Could you check a few things on this drawing? It's one solid part, dimensions in mm from its lowest x, y, z. Coordinates: 2 decimals unless noted, no trailing zeros. Loops run counter-clockwise (first coordinate to the right, second up) from the corner with the lowest first, then second, coordinate; pieces in that order, holes last. Notation, with made-up numbers: M 14,17.25 L 30,17.25 A19 cw 30,31.25 Z; hole C -13.5,19.25 d8. An arc over 180 degrees is marked long. Use one line per item in the form item = value. Start each with the question number.
(1) Imagine slicing it at C-C, the plane y = 7.5. Please give me the cut outline in (x, z) (1 decimal).
(2) Please list where these lines run through material, in increasing order: L1, parallel to Y at x = 16, z = 2.25; L2, parallel to Y at x = 16, z = 4.5; L3, parallel to X at y = 17.5, z = 3.
(3) Thinking about a two-plate mould opening in Y: for the marked faces 1, 2 and 3, which applies, +Y half, -Y half, draft (parallel to the pull), parting line (faces both ways), or undercut?
(4) Imagine slicing it at A-A, the plane y = 16. Please give me the cut outline in (x, z).
(5) Will these pins go through, and if not, where does the flat tip stop? P1, Ø3, axis at x = 27.5, z = 2.5, coming from the -Y side; P2, Ø1.5, axis at y = 14, z = 8, coming from the -X side; P3, Ø5, axis at y = 5, z = 4, coming from the -X side (1 decimal).
(6) Imagine slicing it at D-D, the plane z = 8. Please give me the cut outline in (x, y).
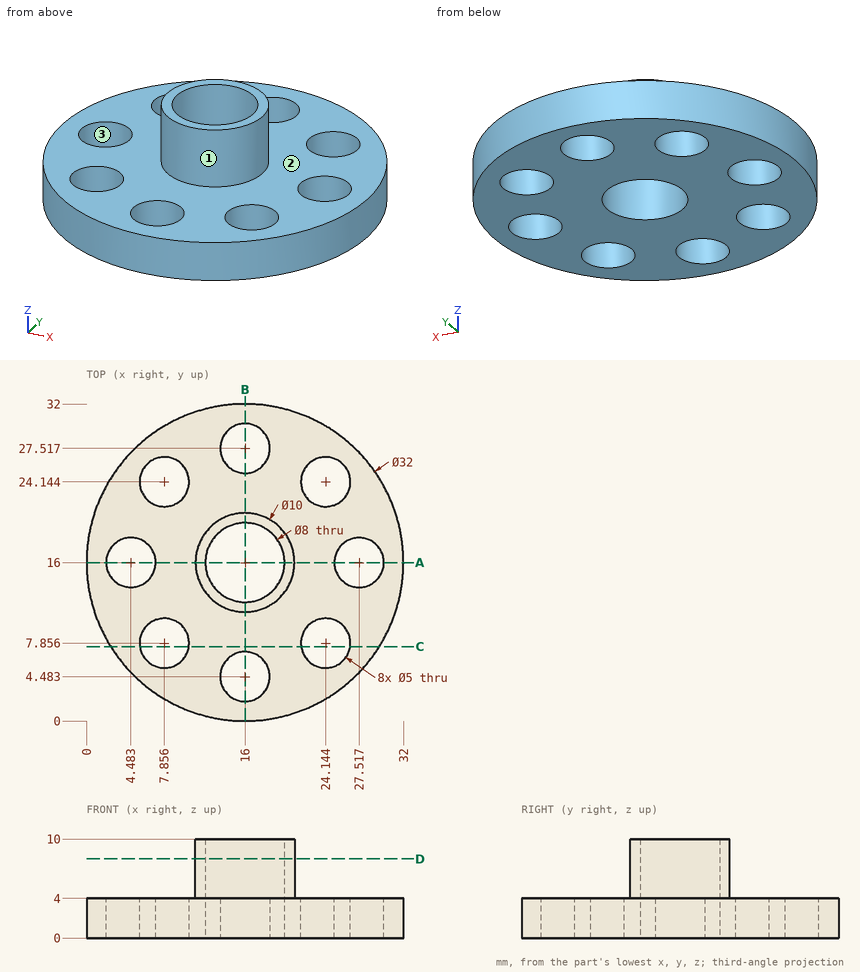
Answer:
q1.outline = M 2.4,0 L 5.4,0 L 5.4,4 L 2.4,4 Z; M 10.3,0 L 21.7,0 L 21.7,4 L 10.3,4 Z; M 26.6,0 L 29.6,0 L 29.6,4 L 26.6,4 Z
q2.L1 = 0 to 1.98, 6.98 to 12, 20 to 25.02, 30.02 to 32
q2.L2 = 11 to 12, 20 to 21
q2.L3 = 0.07 to 2.48, 6.48 to 12.29, 19.71 to 25.52, 29.52 to 31.93
q3.face_1 = parting line
q3.face_2 = draft
q3.face_3 = undercut
q4.outline = M 0,0 L 1.98,0 L 1.98,4 L 0,4 Z; M 6.98,0 L 12,0 L 12,10 L 11,10 L 11,4 L 6.98,4 Z; M 20,0 L 25.02,0 L 25.02,4 L 21,4 L 21,10 L 20,10 Z; M 30.02,0 L 32,0 L 32,4 L 30.02,4 Z
q5.P1 = 3.51
q5.P2 = 11.16
q5.P3 = 2.4
q6.outline = C 16,16 d10; hole C 16,16 d8
